Here's how the part is built. I have some questions about the finished solid (model axes, mm). Face numbers are marked on the shaded views. A direction names the side the tool comes from. Coordinates: 2 decimals unless noted, no trailing zeros. Write each loop counter-clockwise with the first axis right and the second up, starting at its lowest first coordinate (ties: lowest second). Pieces come first, ordered by that corner, then holes. Notation, with made-up numbers: (26, 65.5) -> (78, 65.5) arc R7 ccw to (78, 70.5) -> close; hole circle Ø1 at (11, -35). An arc over 180 degrees is marked (long way). Put each result on its own line as item: value. Start each with the question number.
Item 1: I need wall thicknesses on line 1 (Y direction, x = -79, z = 85); line 2 (Y direction, x = -52, z = 58.95); line 3 (Y direction, x = -78.5, z = 63.5). Which ranges of each line are inside material? Lowest first, please. Write a range as [from, to].
Item 2: I want a section at C-C, the plane x = -52. List the corners of the cut face in (y, z) for me, then the cut area to 3 significant figures.
Item 3: On a 3-axis mill with a long thin cutter (end or side, diameter ignored), from which of +Z, -Z, +X, -X, +Y, -Y can I reach the whole of each face in a straight line? I mean the marked faces 1, 2, 3, 4 and 5. Say none if no direction works.
Item 4: I want a section at B-B, the plane z = 71. List the corners of the cut face in (x, y) for me, then the cut area to 3 significant figures.
Item 5: For pin 1 (11 mm diameter, centred on x = -64, y = -10.5, fed in from +Z); pin 2 (2.5 mm diameter, centred on y = -23, z = 85.5, fed in from +X); pin 3 (3 mm diameter, centred on x = -52, y = -30, fed in from +Z); pin 4 (12 mm diameter, centred on x = -56.5, y = 18, fed in from +Z), each with a flat end and sliding along its axis, tell me the tip position at first contact or that it passes through.
Item 6: I want a section at A-A, the plane y = -22.44. List the corners of the cut face in (x, z) for me.
Item 7: If we mould it in two halves opening along Y, with no side actions, what happens to the marked faces 6, 7 and 8? For each: released by +Y, released by -Y, zero draft, split by the parting line, or undercut.
Item 8: I want a section at D-D, the plane x = -71.5. List the corners of the cut face in (y, z) for me, then the cut area to 3 significant figures.
from build123d import *

# Parameters (mm, degrees)
BASE_4MM_START                          = 57
SKETCH_7_W                              = 36
SKETCH_7_H                              = 68
BASE_4MM_DEPTH                          = 4
TWIN_EAR_SUPPORTS_START                 = 61
SKETCH_8_W                              = 4
SKETCH_8_H                              = 7.7
TWIN_EAR_SUPPORTS_DEPTH                 = 31
INTEGRAL_SHORT_GUSSET_27_4_START        = -27.4
INTEGRAL_SHORT_GUSSET_27_4_DEPTH        = 7.7
INTEGRAL_SHORT_GUSSET_19_7_START        = 19.7
INTEGRAL_SHORT_GUSSET_19_7_DEPTH        = 7.7
BASE_M3_CLEARANCE_START                 = 63
SKETCH_11_R                             = 1.7
BASE_M3_CLEARANCE_DEPTH                 = 7
ACTUAL_CAMERA_44P88_PITCH_M3_DEPTH      = 120
ACTUAL_CAMERA_44P88_PITCH_M3_DEPTH_BACK = 120
SKETCH_12_R                             = 1.7


with BuildPart() as part:
    # Sketch 7 → Base_4mm (new body)
    with BuildSketch(Plane.XY.offset(BASE_4MM_START)):
        with Locations((-66, 0)):
            Rectangle(SKETCH_7_W, SKETCH_7_H)
    extrude(amount=BASE_4MM_DEPTH)

    # Sketch 8 → Twin_ear_supports (add)
    with BuildSketch(Plane.XY.offset(TWIN_EAR_SUPPORTS_START)):
        with Locations((-78, -23.55)):
            Rectangle(SKETCH_8_W, SKETCH_8_H)
        with Locations((-78, 23.55)):
            Rectangle(SKETCH_8_W, SKETCH_8_H)
    extrude(amount=TWIN_EAR_SUPPORTS_DEPTH)

    # Sketch 9 → Integral_short_gusset_-27.4 (add)
    with BuildSketch(Plane(origin=(0, 0, 0), x_dir=(1, 0, 0), z_dir=(0, 1, 0)).offset(INTEGRAL_SHORT_GUSSET_27_4_START)):
        Polygon((-76, -61), (-58, -61), (-76, -74), align=None)
    extrude(amount=INTEGRAL_SHORT_GUSSET_27_4_DEPTH)

    # Sketch 10 → Integral_short_gusset_19.7 (add)
    with BuildSketch(Plane(origin=(0, 0, 0), x_dir=(1, 0, 0), z_dir=(0, 1, 0)).offset(INTEGRAL_SHORT_GUSSET_19_7_START)):
        Polygon((-76, -61), (-58, -61), (-76, -74), align=None)
    extrude(amount=INTEGRAL_SHORT_GUSSET_19_7_DEPTH)

    # Sketch 11 → Base_M3_clearance (cut)
    with BuildSketch(Plane.XY.offset(BASE_M3_CLEARANCE_START)):
        with Locations(Location((-52, -30, 0), (0, 0, 180))):
            Circle(SKETCH_11_R)
        with Locations(Location((-52, 30, 0), (0, 0, 180))):
            Circle(SKETCH_11_R)
    extrude(amount=-BASE_M3_CLEARANCE_DEPTH, mode=Mode.SUBTRACT)

    # Sketch 12 → Actual_camera_44p88_pitch_M3 (cut, two sides: drawn at the far end of the back side and taken through both)
    with BuildSketch(Plane(origin=(0, 0, 0), x_dir=(0, 0, -1), z_dir=(1, 0, 0)).offset(-ACTUAL_CAMERA_44P88_PITCH_M3_DEPTH_BACK)):
        with Locations(Location((-85, -22.44, 0), (0, 0, 180))):
            Circle(SKETCH_12_R)
        with Locations(Location((-85, 22.44, 0), (0, 0, 180))):
            Circle(SKETCH_12_R)
    extrude(amount=ACTUAL_CAMERA_44P88_PITCH_M3_DEPTH + ACTUAL_CAMERA_44P88_PITCH_M3_DEPTH_BACK, mode=Mode.SUBTRACT)


solid = part.part
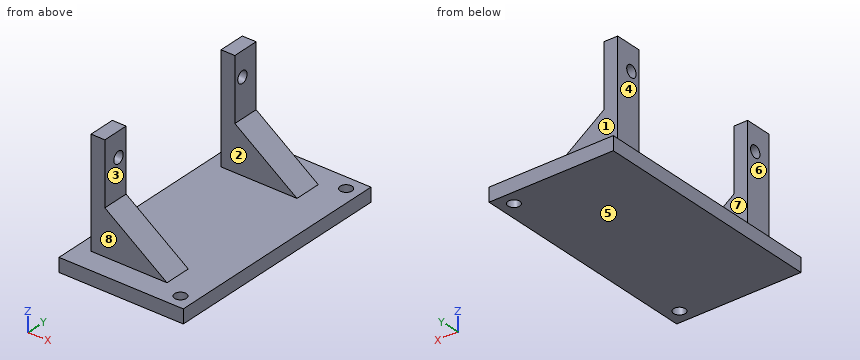
Calculated:
1. line 1: y = [-27.4, -24.14], [-20.74, -19.7], [19.7, 20.74], [24.14, 27.4]
1. line 2: y = [-34, -31.7], [-28.3, 28.3], [31.7, 34]
1. line 3: y = [-27.4, -19.7], [19.7, 27.4]
2. outline: (-34, 57) -> (-31.7, 57) -> (-31.7, 61) -> (-34, 61) -> close; (-28.3, 57) -> (28.3, 57) -> (28.3, 61) -> (-28.3, 61) -> close; (31.7, 57) -> (34, 57) -> (34, 61) -> (31.7, 61) -> close
2. area: 245 mm2
3. face 1: +Z, +X, -X, +Y
3. face 2: +Z, +X, -X
3. face 3: +Z, +X, +Y, -Y
3. face 4: +Z, -X, +Y, -Y
3. face 5: -Z, +X, -X, +Y, -Y
4. outline: (-80, -27.4) -> (-71.85, -27.4) -> (-71.85, -19.7) -> (-80, -19.7) -> close; (-80, 19.7) -> (-71.85, 19.7) -> (-71.85, 27.4) -> (-80, 27.4) -> close
4. area: 126 mm2
5. pin 1: stops at z = 61
5. pin 2: stops at x = -76
5. pin 3: passes through
5. pin 4: stops at z = 64.07
6. outline: (-84, 57) -> (-48, 57) -> (-48, 61) -> (-58, 61) -> (-76, 74) -> (-76, 83.3) -> (-80, 83.3) -> (-80, 61) -> (-84, 61) -> close; (-80, 86.7) -> (-76, 86.7) -> (-76, 92) -> (-80, 92) -> close
7. face 6: zero draft
7. face 7: undercut
7. face 8: released by -Y
8. outline: (-34, 57) -> (34, 57) -> (34, 61) -> (27.4, 61) -> (27.4, 70.75) -> (19.7, 70.75) -> (19.7, 61) -> (-19.7, 61) -> (-19.7, 70.75) -> (-27.4, 70.75) -> (-27.4, 61) -> (-34, 61) -> close
8. area: 422 mm2
